```python
from build123d import *

# Parameters (mm, degrees)
F0_W     = 38.1
F0_H     = 25.4
F1_DEPTH = 12.7
F3_DEPTH = 25.401
F5_DEPTH = 12.8647734687
F6_W     = 25.4
F6_H     = 12.7
F7_DEPTH = 25.4
F9_DEPTH = 25.4


with BuildPart() as f1:
    # F0 (on Front) → F1 (new body, symmetric)
    with BuildSketch(Plane.XZ):
        with Locations((19.05, 12.7)):
            Rectangle(F0_W, F0_H)
    extrude(amount=F1_DEPTH, both=True)

    # F2 (on face) → F3 (cut, through all)
    with BuildSketch(Plane.XY.offset(25.4)):
        Polygon((12.5352265313, -12.7), (19.05, -12.7), (25.2352265313, -12.7), (25.2352265313, 6.35), (12.5352265313, 6.35), align=None)
    extrude(amount=-F3_DEPTH, mode=Mode.SUBTRACT)

    # F4 (on face) → F5 (cut, through all)
    with BuildSketch(Plane.YZ.offset(38.1)):
        Polygon((0, 25.4), (-12.7, 25.4), (-12.7, 12.7), align=None)
    extrude(amount=-F5_DEPTH, mode=Mode.SUBTRACT)

    # F6 (on face) → F7 (cut)
    with BuildSketch(Plane(origin=(0, 0, 0), x_dir=(0, -1, 0), z_dir=(-1, 0, 0))):
        with Locations((0, 19.05)):
            Rectangle(F6_W, F6_H)
    extrude(amount=-F7_DEPTH, mode=Mode.SUBTRACT)

    # F8 (on face) → F9 (cut)
    with BuildSketch(Plane(origin=(0, 0, 0), x_dir=(0, -1, 0), z_dir=(-1, 0, 0))):
        Polygon((0, 12.7), (12.7, 0), (12.7, 12.7), align=None)
    extrude(amount=-F9_DEPTH, mode=Mode.SUBTRACT)


solid = f1.part
```
Source: CAD feature listing. Evaluate the final solid. Frame: model axes, mm. A direction names the side the tool comes from. Coordinates: 2 decimals unless noted, no trailing zeros. Write each loop counter-clockwise with the first axis right and the second up, starting at its lowest first coordinate (ties: lowest second). Pieces come first, ordered by that corner, then holes. Notation, with made-up numbers: (70.5, -21) - (96.5, -21) arc R9 ccw to (96.5, -16) - close; hole circle Ø7 at (16, -7). An arc over 180 degrees is marked (long way). Answer as a JSON object with one key per item and string values.
Q1. Section query A-A, the plane y = -4.75. Output: boundary loops of the cut face in (x, z), plus the area to 3 significant figures.
Ans:
{"outline": "(0, 0) - (12.54, 0) - (12.54, 7.95) - (0, 7.95) - close; (25.24, 0) - (38.1, 0) - (38.1, 20.65) - (25.4, 20.65) - (25.4, 7.95) - (25.24, 7.95) - close", "area": "363 mm2"}
Q2. First-contact query: pin 1 Ø3 at (x, y) = (16, -8) entering from -Z; pin 2 Ø6 at (y, z) = (2, 22) entering from -X; pin 3 Ø4 at (x, z) = (25.5, 16.5) entering from -Y; pin 4 Ø10 at (x, y) = (10, 5) entering from +Z. Flat tips, straight axial feed; report the tip coordinate or a pass-through.
Ans:
{"pin 1": "passes through", "pin 2": "stops at x = 25.4", "pin 3": "stops at y = -10.9", "pin 4": "stops at z = 12.7"}
Q3. Section query C-C, the plane z = 8.75. Output: boundary loops of the cut face in (x, y).
Ans:
{"outline": "(0, -3.95) - (12.54, -3.95) - (12.54, 6.35) - (25.24, 6.35) - (25.24, -3.95) - (25.4, -3.95) - (25.4, -12.7) - (38.1, -12.7) - (38.1, 12.7) - (0, 12.7) - close"}
Q4. Material intervals for line 1 (X direction, y = 4.5, z = 1.25); line 2 (X direction, y = -4.75, z = 11); line 3 (Y direction, x = 15, z = 7), sorted ascending. Write a range as [from, to].
Ans:
{"line 1": "x = [0, 12.54], [25.24, 38.1]", "line 2": "x = [25.4, 38.1]", "line 3": "y = [6.35, 12.7]"}
Q5. Draft query along X for faces 4 (the flat face through (19, 8, 0)), 5 (the flat face through (25.235, -1, 5)), 6 (the flat face through (0, 3, 6)). Return one class per face: released by +X, released by -X, zero draft, split by the parting line, or undercut.
Ans:
{"face 4": "zero draft", "face 5": "undercut", "face 6": "released by -X"}
Q6. Set-up query: faces 1 (the flat face through (6.2, -6.3, 6.4)), 2 (the flat face through (19, 6.35, 6)), 3 (the flat face through (10, 8, 12.7)). Return all of +Z, -Z, +X, -X, +Y, -Y with unobstructed straight access to the full face (end or side cutting, diameter ignored); none if empty.
Ans:
{"face 1": "+Z, -X, -Y", "face 2": "+Z, -Z, -Y", "face 3": "+Z, -X, +Y, -Y"}
Q7. Section query D-D, the plane y = 3.25. Output: boundary loops of the cut face in (x, z).
Ans:
{"outline": "(0, 0) - (12.54, 0) - (12.54, 12.7) - (0, 12.7) - close; (25.24, 0) - (38.1, 0) - (38.1, 25.4) - (25.4, 25.4) - (25.4, 12.7) - (25.24, 12.7) - close"}
Q8. Section query B-B, the plane x = 35.5. Output: boundary loops of the cut face in (y, z), plus the area to 3 significant figures.
Ans:
{"outline": "(-12.7, 0) - (12.7, 0) - (12.7, 25.4) - (0, 25.4) - (-12.7, 12.7) - close", "area": "565 mm2"}
